from build123d import *

# Parameters (mm, degrees)
F0_R      = 55
F1_DEPTH  = 10
F2_R      = 4.1
F3_DEPTH  = 25
F4_R      = 3.1
F5_DEPTH  = 25
F7_D      = 5.5
F7_DEPTH  = 25
F7_TIP    = 1.6523667023
F9_D      = 3.3
F9_DEPTH  = 14.1
F9_TIP    = 0.9914200214
F11_D     = 3.3
F11_DEPTH = 14.1
F11_TIP   = 0.9914200214
F14_D     = 3.3
F14_DEPTH = 14.1
F14_TIP   = 0.9914200214
F15_D     = 3.3
F15_DEPTH = 14.1
F15_TIP   = 0.9914200214


with BuildPart() as f1:
    # F0 (on Top) → F1 (new body)
    with BuildSketch(Plane.XY):
        with BuildLine():
            ThreePointArc((-125, -100), (-117.6776695297, -117.6776695297), (-100, -125))
            Line((-100, -125), (-26.5624980382, -125))
            Line((-26.5624980382, -125), (100.3501711662, -125))
            Line((100.3501711662, -125), (230, -125))
            ThreePointArc((230, -125), (247.6776695297, -117.6776695297), (255, -100))
            Line((255, -100), (255, 100))
            ThreePointArc((255, 100), (247.6776695297, 117.6776695297), (230, 125))
            Line((230, 125), (118.7077554191, 125))
            Line((118.7077554191, 125), (-26.5624980382, 125))
            Line((-26.5624980382, 125), (-100, 125))
            ThreePointArc((-100, 125), (-117.6776695297, 117.6776695297), (-125, 100))
            Line((-125, 100), (-125, -100))
        make_face()
        Circle(F0_R, mode=Mode.SUBTRACT)
    extrude(amount=F1_DEPTH)

    # F2 (on face) → F3 (cut)
    with BuildSketch(Plane.XY.offset(10)):
        with Locations((-45.9619407771, 45.9619407771)):
            Circle(F2_R)
        with Locations((45.9619407771, 45.9619407771)):
            Circle(F2_R)
        with Locations((45.9619407771, -45.9619407771)):
            Circle(F2_R)
        with Locations((-45.9619407771, -45.9619407771)):
            Circle(F2_R)
    extrude(amount=-F3_DEPTH, mode=Mode.SUBTRACT)

    # F4 (on face) → F5 (cut)
    with BuildSketch(Plane.XY.offset(10)):
        with Locations((140, 90)):
            Circle(F4_R)
        with Locations((140, 0)):
            Circle(F4_R)
        with Locations((140, -90)):
            Circle(F4_R)
        with Locations((240, -80)):
            Circle(F4_R)
        with Locations((240, 0)):
            Circle(F4_R)
        with Locations((240, 80)):
            Circle(F4_R)
    extrude(amount=-F5_DEPTH, mode=Mode.SUBTRACT)

    # F7
    with Locations(Plane(origin=(-125, 0, 0), x_dir=(0, -1, 0), z_dir=(-1, 0, 0))):
        with Locations((-66.5, 5), (66.5, 5)):
            Hole(F7_D / 2, depth=F7_DEPTH)
            with Locations((0, 0, -(F7_DEPTH + F7_TIP / 2))):  # 118° drill point
                Cone(0, F7_D / 2, F7_TIP, mode=Mode.SUBTRACT)

    # F9
    with Locations(Plane.XY.offset(10)):
        with Locations((82, 49), (120, 49), (120, -49), (82, -49)):
            Hole(F9_D / 2, depth=F9_DEPTH)
            with Locations((0, 0, -(F9_DEPTH + F9_TIP / 2))):  # 118° drill point
                Cone(0, F9_D / 2, F9_TIP, mode=Mode.SUBTRACT)

    # F11
    with Locations(Plane.XY.offset(10)):
        with Locations((-85, 100), (103, 100)):
            Hole(F11_D / 2, depth=F11_DEPTH)
            with Locations((0, 0, -(F11_DEPTH + F11_TIP / 2))):  # 118° drill point
                Cone(0, F11_D / 2, F11_TIP, mode=Mode.SUBTRACT)

    # F14
    with Locations(Plane.XY.offset(10)):
        with Locations((215, 60), (155, -60)):
            Hole(F14_D / 2, depth=F14_DEPTH)
            with Locations((0, 0, -(F14_DEPTH + F14_TIP / 2))):  # 118° drill point
                Cone(0, F14_D / 2, F14_TIP, mode=Mode.SUBTRACT)

    # F15
    with Locations(Plane(origin=(0, 0, 0), x_dir=(1, 0, 0), z_dir=(0, 0, -1))):
        with Locations((-73.6121593217, -42.5), (-73.6121593217, 42.5), (0, 85), (73.6121593217, 42.5), (73.6121593217, -42.5), (0, -85)):
            Hole(F15_D / 2, depth=F15_DEPTH)
            with Locations((0, 0, -(F15_DEPTH + F15_TIP / 2))):  # 118° drill point
                Cone(0, F15_D / 2, F15_TIP, mode=Mode.SUBTRACT)


solid = f1.part
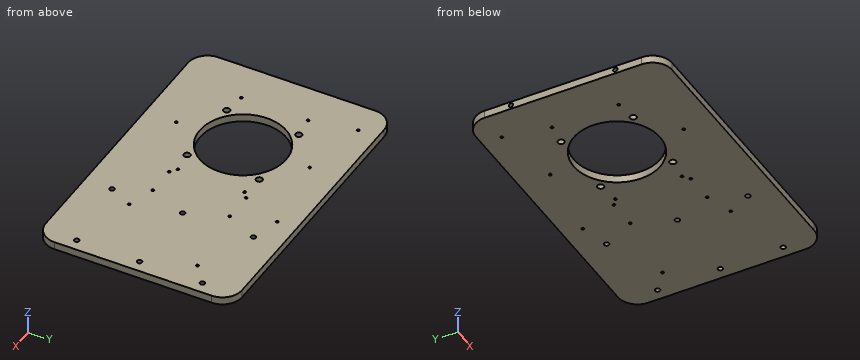
Geometry: final body of the model. Coordinates: model frame, mm. Round coordinates to 2 decimals unless told otherwise and drop trailing zeros. Order: outer loops, then holes, each group sorted by start corner. A loop starts at its lowest first (then second) coordinate and runs counter-clockwise, first axis right, second up. Notation, with made-up numbers: (13.5, 7.25) - (59.5, 7.25) arc R15 cw to (59.5, 20.25) - close; hole circle Ø6 at (77.25, 40). An arc over 180 degrees is marked (long way). Write each question's results on one line, items separated by ' | '.
Item 1: First-contact query: pin 1 Ø6.5 at (x, y) = (45.96, 45.96) entering from +Z; pin 2 Ø3.5 at (y, z) = (66.5, 5) entering from -X. Flat tips, straight axial feed; report the tip coordinate or a pass-through.
Completed:
pin 1: through | pin 2: x = -99.4
Item 2: Section A-A, the plane y = -33. Return the cut outline in (x, z).
Completed:
outline: (-125, 0) - (-44, 0) - (-44, 10) - (-125, 10) - close; (44, 0) - (255, 0) - (255, 10) - (44, 10) - close
Item 3: Section B-B, the plane x = -19. Return the cut outline in (y, z).
Completed:
outline: (-125, 0) - (-51.61, 0) - (-51.61, 10) - (-125, 10) - close; (51.61, 0) - (125, 0) - (125, 10) - (51.61, 10) - close
Item 4: Material intervals for line 1 along Y through (x, z) = (0, 2.5); line 2 along X through (y, z) = (100, 2.25); line 3 along Y through (x, z) = (140, 6.75), sorted ascending. Write a range as [from, to].
Completed:
line 1: [-125, -86.65], [-83.35, -55], [55, 83.35], [86.65, 125] | line 2: [-125, -86.65], [-83.35, 101.35], [104.65, 255] | line 3: [-125, -93.1], [-86.9, -3.1], [3.1, 86.9], [93.1, 125]
